```python
from build123d import *

# Parameters (mm, degrees)
F0_W     = 70
F0_H     = 52
F1_DEPTH = 180
F2_W     = 70
F2_H     = 155
F3_DEPTH = 27
F5_DEPTH = 25
F6_R     = 17.5
F7_DEPTH = 25
F8_R     = 18
F9_DEPTH = 87.001


with BuildPart() as f1:
    # F0 (on Front) → F1 (new body)
    with BuildSketch(Plane.XZ):
        with Locations((-5.444441, 26)):
            Rectangle(F0_W, F0_H)
    extrude(amount=F1_DEPTH)

    # F2 (on face) → F3 (cut)
    with BuildSketch(Plane.XY.offset(52)):
        with Locations((-5.444441, -102.5)):
            Rectangle(F2_W, F2_H)
    extrude(amount=-F3_DEPTH, mode=Mode.SUBTRACT)

    # F4 (on face) → F5 (join)
    with BuildSketch(Plane(origin=(0, 0, 0), x_dir=(-1, 0, 0), z_dir=(0, 1, 0))):
        with BuildLine():
            Line((-29.555559, 52), (40.444441, 52))
            ThreePointArc((40.444441, 52), (5.444441, 87), (-29.555559, 52))
        make_face()
    extrude(amount=-F5_DEPTH)

    # F6 (on Front) → F7 (cut)
    with BuildSketch(Plane.XZ):
        with Locations((-5.444441, 52)):
            Circle(F6_R)
    extrude(amount=F7_DEPTH, mode=Mode.SUBTRACT)

    # F8 (on Top) → F9 (cut, through all)
    with BuildSketch(Plane.XY):
        with Locations((-5.444441, -70)):
            Circle(F8_R)
        with Locations((-5.444441, -135)):
            Circle(F8_R)
    extrude(amount=F9_DEPTH, mode=Mode.SUBTRACT)


solid = f1.part
```
For this review, take the finished solid that the model builds, in its own axes (mm). A direction names the side the tool comes from. Give positions to 0.01 mm unless a question says otherwise; leave off trailing zeros. Loops run counter-clockwise (first coordinate to the right, second up) from the corner with the lowest first, then second, coordinate; pieces in that order, holes last. Notation, with made-up numbers: M 20,16.25 L 74,16.25 A14 ccw 74,23.25 Z; hole C 85,37.5 d7. An arc over 180 degrees is marked long. One line per item, written item: value. Start each with the question number.
Q1. Machinability: for faces 4 (the face through (-6.21, -12.32, 86.99)), 5 (the face through (-5, -25, 70)), which of the approach directions +Z, -Z, +X, -X, +Y, -Y give a long, thin tool a straight path to every point of the face, cutting with its end or side? Answer none if there is none.
Q2. For L1, parallel to X at y = -135, z = 14.75; L2, parallel to Y at x = 9.5, z = 13; L3, parallel to Z at x = 13, y = -170, list the stretches that pass through material, from the lowest coordinate up.
Q3. Add section D-D (z = 55). Give the boundary of the cut face in (x, y), and give its area (3 significant figures).
Q4. Add section A-A (y = -135). Give the boundary of the cut face in (x, z), and give its area (3 significant figures).
Q5. Add section B-B (z = 9). Give the boundary of the cut face in (x, y).
Q6. Clearance check with a flat-ended pin moving along its axis: pin 1 Ø3 at (x, y) = (18, -24) entering from -Z. State where the tip first meets the part, or that it passes through.
Q7. Add section C-C (x = -8). Give the boundary of the cut face in (y, z).
Q8. Draft analysis for pull direction X (two halves, no side actions). For faces 1 (the face through (-6, -101, 25)), 2 (the face through (-40.444, -89, 14)), 3 (the face through (11.247, -12.325, 57.257)), state which applies: released by +X, released by -X, zero draft, split by the parting line, or undercut.
Reply:
1. face 4: +Z, +Y, -Y
1. face 5: +Z, +X, -X, -Y
2. L1: -40.44 to -23.44, 12.56 to 29.56
2. L2: -180 to -145.03, -124.97 to -80.03, -59.97 to 0
2. L3: 0 to 25
3. outline: M -40.32,-25 L -22.69,-25 L -22.69,0 L -40.32,0 Z; M 11.8,-25 L 29.43,-25 L 29.43,0 L 11.8,0 Z
3. area: 882 mm²
4. outline: M -40.44,0 L -23.44,0 L -23.44,25 L -40.44,25 Z; M 12.56,0 L 29.56,0 L 29.56,25 L 12.56,25 Z
4. area: 850 mm²
5. outline: M -40.44,-180 L 29.56,-180 L 29.56,0 L -40.44,0 Z; hole C -5.44,-135 d36; hole C -5.44,-70 d36
6. pin 1: z = 0
7. outline: M -180,0 L -152.82,0 L -152.82,25 L -180,25 Z; M -117.18,0 L -87.82,0 L -87.82,25 L -117.18,25 Z; M -52.18,0 L 0,0 L 0,34.69 L -25,34.69 L -25,25 L -52.18,25 Z; M -25,69.31 L 0,69.31 L 0,86.91 L -25,86.91 Z
8. face 1: zero draft
8. face 2: released by -X
8. face 3: undercut
